Part print with two shaded views. Sizes in mm from the minimum x, y, z corner. Coordinates: 2 decimals unless noted, no trailing zeros. Write each loop counter-clockwise with the first axis right and the second up, starting at its lowest first coordinate (ties: lowest second). Pieces come first, ordered by that corner, then holes. Notation, with made-up numbers: M -4,68 L 49,68 A15 cw 49,74 Z; hole C 47.5,88.25 d4. An arc over 180 degrees is marked long. Answer in a Markdown table with one row per item. Add a question column.
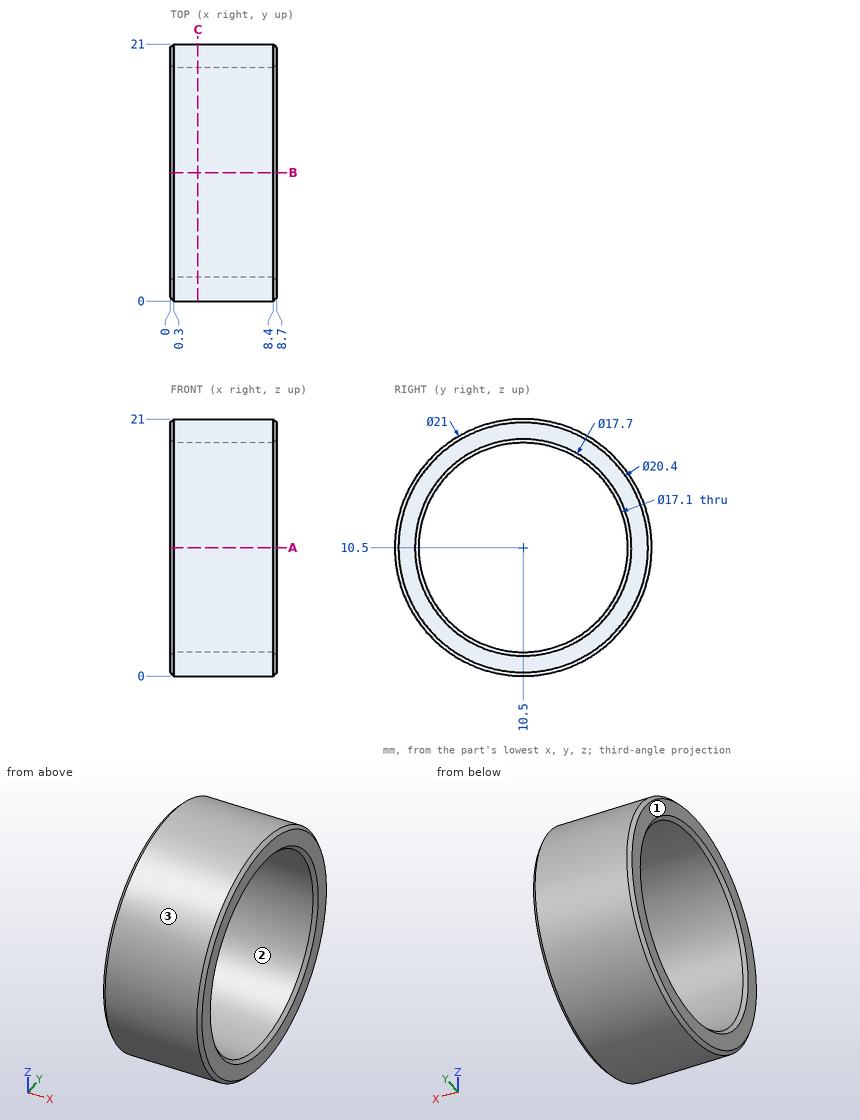
1) Drill centre lines: probe 1 along Z at (x, y) = (2, 10.25); probe 2 along Y at (x, z) = (3.25, 18). Where is each one in solid material? Low to high.
2) Flat gauge pins, fed straight in: pin 1 Ø4 at (x, z) = (1.5, 6.5) entering from +Y; pin 2 Ø2 at (x, y) = (2, 8.5) entering from +Z; pin 3 Ø3 at (x, y) = (3, 13.5) entering from +Z. Where does each tip first touch, or does it go through?
3) Slice it at C-C (x = 2.25). Give the cut face in (y, z).
4) Slice it at A-A (z = 10.5). Give the cut face in (x, y).
5) Two-plate mould, pull along Z, no slides. Class the marked faces 1, 2 and 3: released by +Z, released by -Z, zero draft, split by the parting line, or undercut.
Ans:
| question | item | result |
|---|---|---|
| 1 | probe 1 | z = 0 to 1.95, 19.05 to 21 |
| 1 | probe 2 | y = 3.15 to 6.39, 14.61 to 17.85 |
| 2 | pin 1 | stops at y = 20.81 |
| 2 | pin 2 | stops at z = 20.95 |
| 2 | pin 3 | stops at z = 20.89 |
| 3 | outline | C 10.5,10.5 d21; hole C 10.5,10.5 d17.1 |
| 4 | outline | M 0,0.3 L 0.3,0 L 8.4,0 L 8.7,0.3 L 8.7,1.65 L 8.4,1.95 L 0.3,1.95 L 0,1.65 Z; M 0,19.35 L 0.3,19.05 L 8.4,19.05 L 8.7,19.35 L 8.7,20.7 L 8.4,21 L 0.3,21 L 0,20.7 Z |
| 5 | face 1 | zero draft |
| 5 | face 2 | undercut |
| 5 | face 3 | split by the parting line |
